```python
from build123d import *

# Parameters (mm, degrees)
BOSS_EXTRUDE1_DEPTH     = 14.732
SHELL1_START            = -57.658
SHELL1_OUTLINE_W        = 153.416
SHELL1_OUTLINE_H        = 12.192
SHELL1_DEPTH            = 55.118
CUT_EXTRUDE1_DEPTH      = 103.89414179
CUT_EXTRUDE1_DEPTH_BACK = 103.89414179


# Read off the part's stored shape, not the designer's step: Shell1
with BuildPart() as part:
    # Sketch1 → Boss-Extrude1 (new body)
    with BuildSketch(Plane.XY):
        with BuildLine():
            Line((-79.596309795, 0), (73.819690205, 0))
            ThreePointArc((73.819690205, 0), (75.615741429, -0.743948776), (76.359690205, -2.54))
            Line((76.359690205, -2.54), (76.359690205, -57.658))
            ThreePointArc((76.359690205, -57.658), (75.615741429, -59.454051224), (73.819690205, -60.198))
            Line((73.819690205, -60.198), (-79.596309795, -60.198))
            ThreePointArc((-79.596309795, -60.198), (-81.392361019, -59.454051224), (-82.136309795, -57.658))
            Line((-82.136309795, -57.658), (-82.136309795, -2.54))
            ThreePointArc((-82.136309795, -2.54), (-81.392361019, -0.743948776), (-79.596309795, 0))
        make_face()
    extrude(amount=BOSS_EXTRUDE1_DEPTH)

    # Shell1 outline → Shell1 (cut)
    with BuildSketch(Plane(origin=(0, 0, 0), x_dir=(1, 0, 0), z_dir=(0, 1, 0)).offset(SHELL1_START)):
        with Locations((-2.888309795, -6.096)):
            Rectangle(SHELL1_OUTLINE_W, SHELL1_OUTLINE_H)
    extrude(amount=SHELL1_DEPTH, mode=Mode.SUBTRACT)

    # Sketch3 → Cut-Extrude1 (cut, two sides: drawn at the far end of the back side and taken through both)
    with BuildSketch(Plane(origin=(0, 0, 0), x_dir=(1, 0, 0), z_dir=(0, 1, 0)).offset(-CUT_EXTRUDE1_DEPTH_BACK)):
        Polygon((76.359690205, 0), (0, -11.339454315), (-82.136309795, 0), align=None)
    extrude(amount=CUT_EXTRUDE1_DEPTH + CUT_EXTRUDE1_DEPTH_BACK, mode=Mode.SUBTRACT)


solid = part.part
```
Verification items for the finished model (mm, model axes). A direction names the side the tool comes from. Coordinates: 2 decimals unless noted, no trailing zeros. Loops run counter-clockwise (first coordinate to the right, second up) from the corner with the lowest first, then second, coordinate; pieces in that order, holes last. Notation, with made-up numbers: (43, -12.5) - (93, -12.5) arc R20 cw to (93, 5.5) - close; hole circle Ø7 at (57.25, 25.25). An arc over 180 degrees is marked (long way). Return JSON: item names as keys, results as strings.
1. Section check A-A, the plane y = -37. Record the boundary of the cut face in (x, z).
Established:
{"outline": "(-82.14, 0) - (-79.6, 0.35) - (-79.6, 12.19) - (73.82, 12.19) - (73.82, 0.38) - (76.36, 0) - (76.36, 14.73) - (-82.14, 14.73) - close"}
2. Section check C-C, the plane x = -7.5. Record the boundary of the cut face in (y, z), then the cut area to 3 significant figures.
Established:
{"outline": "(-60.2, 10.3) - (-57.66, 10.3) - (-57.66, 12.19) - (-2.54, 12.19) - (-2.54, 10.3) - (0, 10.3) - (0, 14.73) - (-60.2, 14.73) - close", "area": "162 mm2"}
3. Tool access check on faces 1 (the flat face through (75.124, -30.239, 0.184)), 2 (the flat face through (-82.136, -30, 7)), 3 (the flat face through (-4, -2.54, 11)). Record the directions out of +Z, -Z, +X, -X, +Y, -Y that give a thin tool (end or side, any length) a straight path to the whole face; none if there is none.
Established:
{"face 1": "-Z, +Y, -Y", "face 2": "+Z, -Z, -X, +Y, -Y", "face 3": "-Z"}
4. Thickness scan on L1, parallel to X at y = -37.5, z = 11.25; L2, parallel to Y at x = -65.5, z = 12; L3, parallel to Z at x = -51.5, y = -32.5. Record the ranges inside material, lowest first.
Established:
{"L1": "x = -82.14 to -79.6, 73.82 to 76.36", "L2": "y = -60.2 to -57.66, -2.54 to 0", "L3": "z = 12.19 to 14.73"}
5. Section check B-B, the plane z = 4.5. Record the boundary of the cut face in (x, y).
Established:
{"outline": "(-82.14, -57.66) arc R2.54 ccw to (-79.6, -60.2) - (-49.54, -60.2) - (-49.54, -57.66) - (-79.6, -57.66) - (-79.6, -2.54) - (-49.54, -2.54) - (-49.54, 0) - (-79.6, 0) arc R2.54 ccw to (-82.14, -2.54) - close; (46.06, -60.2) - (73.82, -60.2) arc R2.54 ccw to (76.36, -57.66) - (76.36, -2.54) arc R2.54 ccw to (73.82, 0) - (46.06, 0) - (46.06, -2.54) - (73.82, -2.54) - (73.82, -57.66) - (46.06, -57.66) - close"}
6. Go/stop test with flat-tipped pins: pin 1 (4 mm diameter, centred on x = 3, y = -18, fed in from -Z); pin 2 (1.5 mm diameter, centred on x = -14.5, z = 7.5, fed in from -Y). Record where each tip stops, or that it passes through.
Established:
{"pin 1": "stops at z = 12.19", "pin 2": "passes through"}
7. Mould release check, pull along Y, two halves, no side actions. Record for faces 4 (the flat face through (-2, -60.198, 12)), 5 (the flat face through (-4, -57.658, 11)), 6 (the flat face through (-4, 0, 12)), 7 (the flat face through (-2, -30, 14.732)): +Y half, -Y half, draft (parallel to the pull), parting line (faces both ways), or undercut.
Established:
{"face 4": "-Y half", "face 5": "undercut", "face 6": "+Y half", "face 7": "draft"}
